Check sheet for the drawn part. Datum: minimum x, y, z corner. Units: mm. Give positions to 0.01 mm unless a question says otherwise; leave off trailing zeros. Write each loop counter-clockwise with the first axis right and the second up, starting at its lowest first coordinate (ties: lowest second). Pieces come first, ordered by that corner, then holes. Notation, with made-up numbers: (-24.5, -20.5) -> (10.5, -20.5) arc R15 ccw to (10.5, -6.5) -> close; hole circle Ø7 at (29.25, -31.5). An arc over 180 degrees is marked (long way). Answer as CSV lines item,"result". Start each with the question number.
1) Material ranges on L1, parallel to Y at x = 34, z = 2.4; L2, parallel to X at y = 4, z = 1.7; L3, parallel to Y at x = 52, z = 0.85, recorded low to high.
2) Sectioned sample at C-C on x = 47. Record the cut outline in (y, z), and give its area (3 significant figures).
3) Sectioned sample at D-D on y = 9. Record the cut outline in (x, z), and give its area (3 significant figures).
4) Sectioned sample at B-B on y = 3.6. Record the cut outline in (x, z), and give its area (3 significant figures).
5) Sectioned sample at A-A on z = 2.5. Give the number of separate pieces and of enclosed holes in the cut face, and give its area (3 significant figures).
6) Gauge pin test, flat end, axial feed: pin 1 Ø3 at (x, y) = (26, 44) entering from -Z. Record the tip position at first contact, or that the pin passes through.
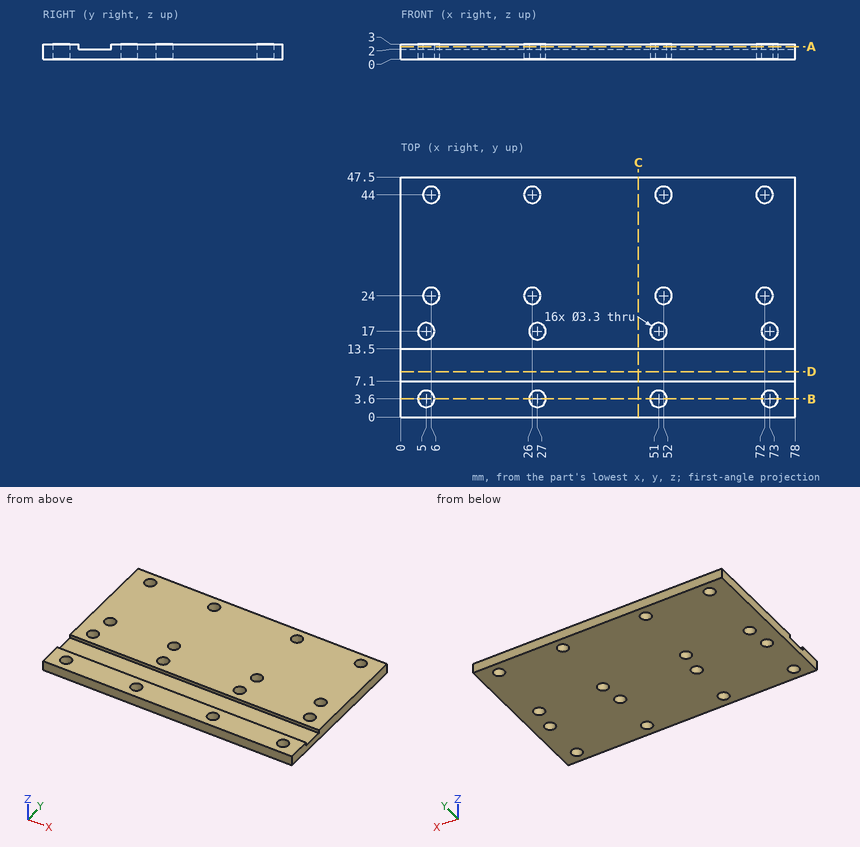
Ans:
1,L1,"y = 0 to 7.1, 13.5 to 47.5"
1,L2,"x = 0 to 3.4, 6.6 to 25.4, 28.6 to 49.4, 52.6 to 71.4, 74.6 to 78"
1,L3,"y = 0 to 2.29, 4.91 to 15.69, 18.31 to 22.35, 25.65 to 42.35, 45.65 to 47.5"
2,outline,"(0, 0) -> (47.5, 0) -> (47.5, 3) -> (13.5, 3) -> (13.5, 2) -> (7.1, 2) -> (7.1, 3) -> (0, 3) -> close"
2,area,"136 mm²"
3,outline,"(0, 0) -> (78, 0) -> (78, 2) -> (0, 2) -> close"
3,area,"156 mm²"
4,outline,"(0, 0) -> (3.35, 0) -> (3.35, 3) -> (0, 3) -> close; (6.65, 0) -> (25.35, 0) -> (25.35, 3) -> (6.65, 3) -> close; (28.65, 0) -> (49.35, 0) -> (49.35, 3) -> (28.65, 3) -> close; (52.65, 0) -> (71.35, 0) -> (71.35, 3) -> (52.65, 3) -> close; (74.65, 0) -> (78, 0) -> (78, 3) -> (74.65, 3) -> close"
4,area,"194 mm²"
5,separate pieces,"2"
5,enclosed holes,"16"
5,area,"3,070 mm²"
6,pin 1,"passes through"
